Autodesk Fusion 360 part; units mm, degrees
sketch "Boceto1" plane through (0, 0, 0) normal (0, 1, 0) x (1, 0, 0)
  line L0 (0, 0) -> (4, 0)
  line L1 (4, 0) -> (4, 100)
  line L2 (4, 100) -> (0, 100)
  line L3 (0, 100) -> (0, 0)
  dimension "d1" = 4
  dimension "d2" = 100
extrude "Extruir1" add sketch "Boceto1" along normal blind 50
sketch "Boceto2" plane through (4, 0, 0) normal (1, 0, 0) x (0, 0, -1)
  line L0 (0, 0) -> (100, 0)
  line L1 (100, 0) -> (100, 50)
  line L2 (100, 50) -> (0, 50)
  line L3 (0, 50) -> (0, 0)
  line L4 (0, 0) -> (0, 7.5)
  line L5 (0, 7.5) -> (22.5, 7.5)
  line L6 (22.5, 7.5) -> (77.5, 7.5)
  line L7 (77.5, 7.5) -> (77.5, 42.5)
  line L8 (77.5, 42.5) -> (22.5, 42.5)
  circle A0 centre (22.5, 42.5) radius 1.5
  circle A1 centre (77.5, 42.5) radius 1.5
  circle A2 centre (22.5, 7.5) radius 1.5
  circle A3 centre (77.5, 7.5) radius 1.5
  line L9 (0, 50) -> (4, 50)
  line L10 (4, 50) -> (4, 46)
  line L11 (4, 46) -> (96, 46)
  line L12 (96, 46) -> (96, 4)
  line L13 (96, 4) -> (4, 4)
  line L14 (4, 4) -> (4, 46)
  line L15 (50, 46) -> (50, 25)
  line L16 (47.1132, 30) -> (44.2265, 25)
  line L17 (44.2265, 25) -> (47.1132, 20)
  line L18 (47.1132, 20) -> (52.8868, 20)
  line L19 (52.8868, 20) -> (55.7735, 25)
  line L20 (55.7735, 25) -> (52.8868, 30)
  line L21 (52.8868, 30) -> (47.1132, 30)
  line L22 (9.1132, 30) -> (6.2265, 25)
  line L23 (9.1132, 20) -> (14.8868, 20)
  line L24 (14.8868, 20) -> (17.7735, 25)
  line L25 (6.2265, 25) -> (9.1132, 20)
  line L26 (17.7735, 25) -> (14.8868, 30)
  line L27 (14.8868, 30) -> (9.1132, 30)
  line L28 (28.1132, 30) -> (25.2265, 25)
  line L29 (28.1132, 20) -> (33.8868, 20)
  line L30 (33.8868, 20) -> (36.7735, 25)
  line L31 (25.2265, 25) -> (28.1132, 20)
  line L32 (36.7735, 25) -> (33.8868, 30)
  line L33 (33.8868, 30) -> (28.1132, 30)
  line L34 (66.1132, 30) -> (63.2265, 25)
  line L35 (66.1132, 20) -> (71.8868, 20)
  line L36 (71.8868, 20) -> (74.7735, 25)
  line L37 (63.2265, 25) -> (66.1132, 20)
  line L38 (74.7735, 25) -> (71.8868, 30)
  line L39 (71.8868, 30) -> (66.1132, 30)
  line L40 (85.1132, 30) -> (82.2265, 25)
  line L41 (85.1132, 20) -> (90.8868, 20)
  line L42 (90.8868, 20) -> (93.7735, 25)
  line L43 (82.2265, 25) -> (85.1132, 20)
  line L44 (93.7735, 25) -> (90.8868, 30)
  line L45 (90.8868, 30) -> (85.1132, 30)
  line L46 (17.7735, 12) -> (14.8868, 17)
  line L47 (85.1132, 17) -> (82.2265, 12)
  line L48 (14.8868, 17) -> (9.1132, 17)
  line L49 (90.8868, 7) -> (93.7735, 12)
  line L50 (47.1132, 7) -> (52.8868, 7)
  line L51 (28.1132, 17) -> (25.2265, 12)
  line L52 (47.1132, 17) -> (44.2265, 12)
  line L53 (85.1132, 7) -> (90.8868, 7)
  line L54 (52.8868, 7) -> (55.7735, 12)
  line L55 (63.2265, 12) -> (66.1132, 7)
  line L56 (9.1132, 7) -> (14.8868, 7)
  line L57 (14.8868, 7) -> (17.7735, 12)
  line L58 (52.8868, 17) -> (47.1132, 17)
  line L59 (74.7735, 12) -> (71.8868, 17)
  line L60 (28.1132, 7) -> (33.8868, 7)
  line L61 (36.7735, 12) -> (33.8868, 17)
  line L62 (82.2265, 12) -> (85.1132, 7)
  line L63 (71.8868, 17) -> (66.1132, 17)
  line L64 (33.8868, 17) -> (28.1132, 17)
  line L65 (93.7735, 12) -> (90.8868, 17)
  line L66 (9.1132, 17) -> (6.2265, 12)
  line L67 (33.8868, 7) -> (36.7735, 12)
  line L68 (25.2265, 12) -> (28.1132, 7)
  line L69 (71.8868, 7) -> (74.7735, 12)
  line L70 (55.7735, 12) -> (52.8868, 17)
  line L71 (6.2265, 12) -> (9.1132, 7)
  line L72 (66.1132, 7) -> (71.8868, 7)
  line L73 (66.1132, 17) -> (63.2265, 12)
  line L74 (44.2265, 12) -> (47.1132, 7)
  line L75 (90.8868, 17) -> (85.1132, 17)
  line L76 (17.7735, 38) -> (14.8868, 43)
  line L77 (85.1132, 43) -> (82.2265, 38)
  line L78 (14.8868, 43) -> (9.1132, 43)
  line L79 (90.8868, 33) -> (93.7735, 38)
  line L80 (47.1132, 33) -> (52.8868, 33)
  line L81 (28.1132, 43) -> (25.2265, 38)
  line L82 (47.1132, 43) -> (44.2265, 38)
  line L83 (85.1132, 33) -> (90.8868, 33)
  line L84 (52.8868, 33) -> (55.7735, 38)
  line L85 (63.2265, 38) -> (66.1132, 33)
  line L86 (9.1132, 33) -> (14.8868, 33)
  line L87 (14.8868, 33) -> (17.7735, 38)
  line L88 (52.8868, 43) -> (47.1132, 43)
  line L89 (74.7735, 38) -> (71.8868, 43)
  line L90 (28.1132, 33) -> (33.8868, 33)
  line L91 (36.7735, 38) -> (33.8868, 43)
  line L92 (82.2265, 38) -> (85.1132, 33)
  line L93 (71.8868, 43) -> (66.1132, 43)
  line L94 (33.8868, 43) -> (28.1132, 43)
  line L95 (93.7735, 38) -> (90.8868, 43)
  line L96 (9.1132, 43) -> (6.2265, 38)
  line L97 (33.8868, 33) -> (36.7735, 38)
  line L98 (25.2265, 38) -> (28.1132, 33)
  line L99 (71.8868, 33) -> (74.7735, 38)
  line L100 (55.7735, 38) -> (52.8868, 43)
  line L101 (6.2265, 38) -> (9.1132, 33)
  line L102 (66.1132, 33) -> (71.8868, 33)
  line L103 (66.1132, 43) -> (63.2265, 38)
  line L104 (44.2265, 38) -> (47.1132, 33)
  line L105 (90.8868, 43) -> (85.1132, 43)
  point P0 (50, 25)
  point P1 (12, 25)
  point P2 (12, 25)
  point P3 (31, 25)
  point P4 (31, 25)
  point P5 (69, 25)
  point P6 (69, 25)
  point P7 (88, 25)
  point P8 (88, 25)
  point P9 (12, 12)
  point P10 (50, 12)
  point P11 (69, 12)
  point P12 (31, 12)
  point P13 (88, 12)
  point P14 (50, 12)
  point P15 (31, 12)
  point P16 (88, 12)
  point P17 (69, 12)
  point P18 (12, 12)
  point P19 (12, 38)
  point P20 (50, 38)
  point P21 (69, 38)
  point P22 (31, 38)
  point P23 (88, 38)
  point P24 (50, 38)
  point P25 (31, 38)
  point P26 (88, 38)
  point P27 (69, 38)
  point P28 (12, 38)
  dimension "d5" = 7.5
  dimension "d6" = 22.5
  dimension "d7" = 55
  dimension "d8" = 35
  dimension "d9" = 3
  dimension "d10" = 3
  dimension "d11" = 3
  dimension "d12" = 3
  dimension "d13" = 4
  dimension "d14" = 4
  dimension "d15" = 92
  dimension "d16" = 42
  dimension "d17" = 5
  dimension "d20" = 38
  dimension "d21" = 0
  dimension "d24" = 0
  dimension "d25" = 13
extrude "Extruir2" cut sketch "Boceto2" against normal blind 13 contours L16 L17 L18 L19 L20 L21 | A0 | L8 L81 L90 L91 L97 L98 | L8 L81 L91 L94 | L5 L46 L48 L57 L66 L71 | L5 L56 L57 L71 | L5 L6 A2 | L5 L6 A2 | L8 L15 L88 L100 | L8 L15 L82 L88 | L8 L15 L80 L82 L104 | L8 L15 L80 L84 L100 | L6 L51 L61 L64 L67 L68 | L6 L60 L67 L68 | L8 L89 L93 L103 | L8 L85 L89 L99 L102 L103 | L6 L52 L54 L58 L70 L74 | L6 L50 L54 L74 | L7 L8 A1 | L7 L8 A1 | L6 L55 L59 L63 L69 L73 | L6 L55 L69 L72 | L6 L7 A3 | L6 L7 A3 | L22 L23 L24 L25 L26 L27 | L28 L29 L30 L31 L32 L33 | L34 L35 L36 L37 L38 L39 | L40 L41 L42 L43 L44 L45 | L47 L49 L53 L62 L65 L75 | L76 L78 L86 L87 L96 L101 | L77 L79 L83 L92 L95 L105
sketch "Boceto3" plane through (4, 0, 0) normal (1, 0, 0) x (0, 0, -1)
  line L0 (52.8868, 7) -> (47.1132, 7)
  line L1 (47.1132, 7) -> (44.2265, 12)
  line L2 (44.2265, 12) -> (47.1132, 17)
  line L3 (47.1132, 17) -> (52.8868, 17)
  line L4 (52.8868, 17) -> (55.7735, 12)
  line L5 (55.7735, 12) -> (52.8868, 7)
  line L6 (14.8868, 33) -> (9.1132, 33)
  line L7 (9.1132, 33) -> (6.2265, 38)
  line L8 (6.2265, 38) -> (9.1132, 43)
  line L9 (9.1132, 43) -> (14.8868, 43)
  line L10 (14.8868, 43) -> (17.7735, 38)
  line L11 (17.7735, 38) -> (14.8868, 33)
  line L12 (63.2265, 25) -> (66.1132, 30)
  line L13 (66.1132, 30) -> (71.8868, 30)
  line L14 (71.8868, 30) -> (74.7735, 25)
  line L15 (74.7735, 25) -> (71.8868, 20)
  line L16 (71.8868, 20) -> (66.1132, 20)
  line L17 (66.1132, 20) -> (63.2265, 25)
  circle A0 centre (77.5, 42.5) radius 1.5
  circle A1 centre (22.5, 42.5) radius 1.5
  line L18 (66.1132, 33) -> (63.2265, 38)
  line L19 (63.2265, 38) -> (66.1132, 43)
  line L20 (66.1132, 43) -> (71.8868, 43)
  line L21 (71.8868, 43) -> (74.7735, 38)
  line L22 (74.7735, 38) -> (71.8868, 33)
  line L23 (71.8868, 33) -> (66.1132, 33)
  line L24 (82.2265, 12) -> (85.1132, 17)
  line L25 (85.1132, 17) -> (90.8868, 17)
  line L26 (90.8868, 17) -> (93.7735, 12)
  line L27 (93.7735, 12) -> (90.8868, 7)
  line L28 (90.8868, 7) -> (85.1132, 7)
  line L29 (85.1132, 7) -> (82.2265, 12)
  line L30 (6.2265, 25) -> (9.1132, 30)
  line L31 (9.1132, 30) -> (14.8868, 30)
  line L32 (14.8868, 30) -> (17.7735, 25)
  line L33 (17.7735, 25) -> (14.8868, 20)
  line L34 (14.8868, 20) -> (9.1132, 20)
  line L35 (9.1132, 20) -> (6.2265, 25)
  line L36 (33.8868, 7) -> (28.1132, 7)
  line L37 (28.1132, 7) -> (25.2265, 12)
  line L38 (25.2265, 12) -> (28.1132, 17)
  line L39 (28.1132, 17) -> (33.8868, 17)
  line L40 (33.8868, 17) -> (36.7735, 12)
  line L41 (36.7735, 12) -> (33.8868, 7)
  line L42 (66.1132, 7) -> (63.2265, 12)
  line L43 (63.2265, 12) -> (66.1132, 17)
  line L44 (66.1132, 17) -> (71.8868, 17)
  line L45 (71.8868, 17) -> (74.7735, 12)
  line L46 (74.7735, 12) -> (71.8868, 7)
  line L47 (71.8868, 7) -> (66.1132, 7)
  line L48 (14.8868, 7) -> (9.1132, 7)
  line L49 (9.1132, 7) -> (6.2265, 12)
  line L50 (6.2265, 12) -> (9.1132, 17)
  line L51 (9.1132, 17) -> (14.8868, 17)
  line L52 (14.8868, 17) -> (17.7735, 12)
  line L53 (17.7735, 12) -> (14.8868, 7)
  line L54 (44.2265, 25) -> (47.1132, 30)
  line L55 (47.1132, 30) -> (52.8868, 30)
  line L56 (52.8868, 30) -> (55.7735, 25)
  line L57 (55.7735, 25) -> (52.8868, 20)
  line L58 (52.8868, 20) -> (47.1132, 20)
  line L59 (47.1132, 20) -> (44.2265, 25)
  line L60 (82.2265, 38) -> (85.1132, 43)
  line L61 (85.1132, 43) -> (90.8868, 43)
  line L62 (90.8868, 43) -> (93.7735, 38)
  line L63 (93.7735, 38) -> (90.8868, 33)
  line L64 (90.8868, 33) -> (85.1132, 33)
  line L65 (85.1132, 33) -> (82.2265, 38)
  line L66 (33.8868, 33) -> (28.1132, 33)
  line L67 (28.1132, 33) -> (25.2265, 38)
  line L68 (25.2265, 38) -> (28.1132, 43)
  line L69 (28.1132, 43) -> (33.8868, 43)
  line L70 (33.8868, 43) -> (36.7735, 38)
  line L71 (36.7735, 38) -> (33.8868, 33)
  line L72 (52.8868, 33) -> (47.1132, 33)
  line L73 (47.1132, 33) -> (44.2265, 38)
  line L74 (44.2265, 38) -> (47.1132, 43)
  line L75 (47.1132, 43) -> (52.8868, 43)
  line L76 (52.8868, 43) -> (55.7735, 38)
  line L77 (55.7735, 38) -> (52.8868, 33)
  line L78 (82.2265, 25) -> (85.1132, 30)
  line L79 (85.1132, 30) -> (90.8868, 30)
  line L80 (90.8868, 30) -> (93.7735, 25)
  line L81 (93.7735, 25) -> (90.8868, 20)
  line L82 (90.8868, 20) -> (85.1132, 20)
  line L83 (85.1132, 20) -> (82.2265, 25)
  line L84 (25.2265, 25) -> (28.1132, 30)
  line L85 (28.1132, 30) -> (33.8868, 30)
  line L86 (33.8868, 30) -> (36.7735, 25)
  line L87 (36.7735, 25) -> (33.8868, 20)
  line L88 (33.8868, 20) -> (28.1132, 20)
  line L89 (28.1132, 20) -> (25.2265, 25)
  circle A2 centre (22.5, 7.5) radius 1.5
  circle A3 centre (77.5, 7.5) radius 1.5
  line L90 (0, 0) -> (100, 0)
  line L91 (100, 0) -> (100, 50)
  line L92 (100, 50) -> (0, 50)
  line L93 (0, 50) -> (0, 0)
The model under review builds one solid part; all positions refer to its coordinate system, in mm. Give positions to 0.01 mm unless a question says otherwise; leave off trailing zeros. Write each loop counter-clockwise with the first axis right and the second up, starting at its lowest first coordinate (ties: lowest second). Pieces come first, ordered by that corner, then holes. Notation, with made-up numbers: M -17,-19 L 27,-19 A24 ccw 27,-8 Z; hole C -33,79 d5. An arc over 180 degrees is marked long. One line per question, with ' | ' between items. Start each with the question number.
Item 1: Wall thickness on line 1 (Y direction, x = 2.3, z = -22.5); line 2 (Z direction, x = 1.6, y = 12); line 3 (Y direction, x = 3.45, z = -26): over which ranges is each line inside the solid? List them lowest first. Write a range as from..to.
Item 2: We need section B-B on y = 15. Write out the cut boundary in (x, z), plus the area to 3 significant figures.
Item 3: We need section A-A on z = -77.5. Write out the cut boundary in (x, y).
Item 4: We need section C-C on x = 1.7. Give the number of separate pieces and of enclosed holes in the cut face, plus the area to 3 significant figures.
Results found:
1) line 1: y = 0..6, 9..41, 44..50 | line 2: z = -100..-93.77, -82.23..-74.77, -63.23..-55.77, -44.23..-36.77, -25.23..-17.77, -6.23..0 | line 3: y = 0..10.66, 13.34..23.66, 26.34..36.66, 39.34..50
2) outline: M 0,-100 L 4,-100 L 4,-92.04 L 0,-92.04 Z; M 0,-83.96 L 4,-83.96 L 4,-73.04 L 0,-73.04 Z; M 0,-64.96 L 4,-64.96 L 4,-54.04 L 0,-54.04 Z; M 0,-45.96 L 4,-45.96 L 4,-35.04 L 0,-35.04 Z; M 0,-26.96 L 4,-26.96 L 4,-16.04 L 0,-16.04 Z; M 0,-7.96 L 4,-7.96 L 4,0 L 0,0 Z | area: 238 mm2
3) outline: M 0,0 L 4,0 L 4,6 L 0,6 Z; M 0,9 L 4,9 L 4,41 L 0,41 Z; M 0,44 L 4,44 L 4,50 L 0,50 Z
4) separate pieces: 1 | enclosed holes: 19 | area: 3,670 mm2
